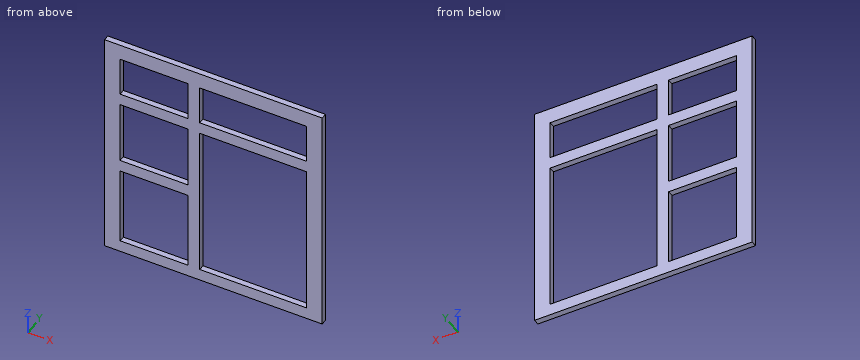
from build123d import *

# Parameters (mm, degrees)
F0_W     = 349.25
F0_H     = 38.1
F0_W_2   = 222.25
F1_DEPTH = 19.05


with BuildPart() as f1:
    # F0 (on Front) → F1 (new body)
    with BuildSketch(Plane.XZ):
        Polygon((0, 749.3), (0, 0), (50.8, 0), (50.8, 38.1), (50.8, 292.1), (50.8, 330.2), (50.8, 533.4), (50.8, 571.5), (50.8, 698.5), (50.8, 749.3), align=None)
        Polygon((660.4, 749.3), (50.8, 749.3), (50.8, 698.5), (273.05, 698.5), (311.15, 698.5), (660.4, 698.5), align=None)
        Polygon((660.4, 38.1), (660.4, 0), (711.2, 0), (711.2, 749.3), (660.4, 749.3), (660.4, 698.5), (660.4, 571.5), (660.4, 533.4), align=None)
        Polygon((273.05, 292.1), (273.05, 38.1), (311.15, 38.1), (311.15, 533.4), (311.15, 571.5), (311.15, 698.5), (273.05, 698.5), (273.05, 571.5), (273.05, 533.4), (273.05, 330.2), align=None)
        with Locations((485.775, 552.45)):
            Rectangle(F0_W, F0_H)
        with Locations((161.925, 552.45)):
            Rectangle(F0_W_2, F0_H)
        with Locations((161.925, 311.15)):
            Rectangle(F0_W_2, F0_H)
        Polygon((50.8, 38.1), (50.8, 0), (660.4, 0), (660.4, 38.1), (311.15, 38.1), (273.05, 38.1), align=None)
    extrude(amount=F1_DEPTH)


solid = f1.part
Check sheet for the modelled part. Datum: model origin and axes. Units: mm. Round coordinates to 2 decimals unless told otherwise and drop trailing zeros. Loops run counter-clockwise (first coordinate to the right, second up) from the corner with the lowest first, then second, coordinate; pieces in that order, holes last.
1. Sectioned sample at B-B on y = -9.25. Record the boundary of the cut face in (x, z).
2. Sectioned sample at C-C on x = 624. Record the boundary of the cut face in (y, z), and give its area (3 significant figures).
3. Sectioned sample at D-D on z = 635.5. Record the boundary of the cut face in (x, y).
4. Scan lines: probe 1 along Z at (x, y) = (487, -5); probe 2 along X at (y, z) = (-14.25, 683); probe 3 along Z at (x, y) = (271, -4). Record each from-to range of solid material in increasing order.
5. Sectioned sample at A-A on x = 75.5. Record the boundary of the cut face in (y, z).
Recorded:
1. outline: (0, 0) - (711.2, 0) - (711.2, 749.3) - (0, 749.3) - close; hole (50.8, 38.1) - (273.05, 38.1) - (273.05, 292.1) - (50.8, 292.1) - close; hole (50.8, 330.2) - (273.05, 330.2) - (273.05, 533.4) - (50.8, 533.4) - close; hole (50.8, 571.5) - (273.05, 571.5) - (273.05, 698.5) - (50.8, 698.5) - close; hole (311.15, 38.1) - (660.4, 38.1) - (660.4, 533.4) - (311.15, 533.4) - close; hole (311.15, 571.5) - (660.4, 571.5) - (660.4, 698.5) - (311.15, 698.5) - close
2. outline: (-19.05, 0) - (0, 0) - (0, 38.1) - (-19.05, 38.1) - close; (-19.05, 533.4) - (0, 533.4) - (0, 571.5) - (-19.05, 571.5) - close; (-19.05, 698.5) - (0, 698.5) - (0, 749.3) - (-19.05, 749.3) - close
2. area: 2,420 mm2
3. outline: (0, -19.05) - (50.8, -19.05) - (50.8, 0) - (0, 0) - close; (273.05, -19.05) - (311.15, -19.05) - (311.15, 0) - (273.05, 0) - close; (660.4, -19.05) - (711.2, -19.05) - (711.2, 0) - (660.4, 0) - close
4. probe 1: z = 0 to 38.1, 533.4 to 571.5, 698.5 to 749.3
4. probe 2: x = 0 to 50.8, 273.05 to 311.15, 660.4 to 711.2
4. probe 3: z = 0 to 38.1, 292.1 to 330.2, 533.4 to 571.5, 698.5 to 749.3
5. outline: (-19.05, 0) - (0, 0) - (0, 38.1) - (-19.05, 38.1) - close; (-19.05, 292.1) - (0, 292.1) - (0, 330.2) - (-19.05, 330.2) - close; (-19.05, 533.4) - (0, 533.4) - (0, 571.5) - (-19.05, 571.5) - close; (-19.05, 698.5) - (0, 698.5) - (0, 749.3) - (-19.05, 749.3) - close
